Here's the drawing with two shaded views (mm, measured from the low corner). I have some questions. Coordinates: 2 decimals unless noted, no trailing zeros. Order: outer loops, then holes, each group sorted by start corner. A loop starts at its lowest first (then second) coordinate and runs counter-clockwise, first axis right, second up. Notation, with made-up numbers: (44, -22.5) -> (100, -22.5) arc R25 cw to (100, 1.5) -> close; hole circle Ø6 at (66.5, -24). An arc over 180 degrees is marked (long way). Return JSON: item names as keys, results as strings. Group by question number.
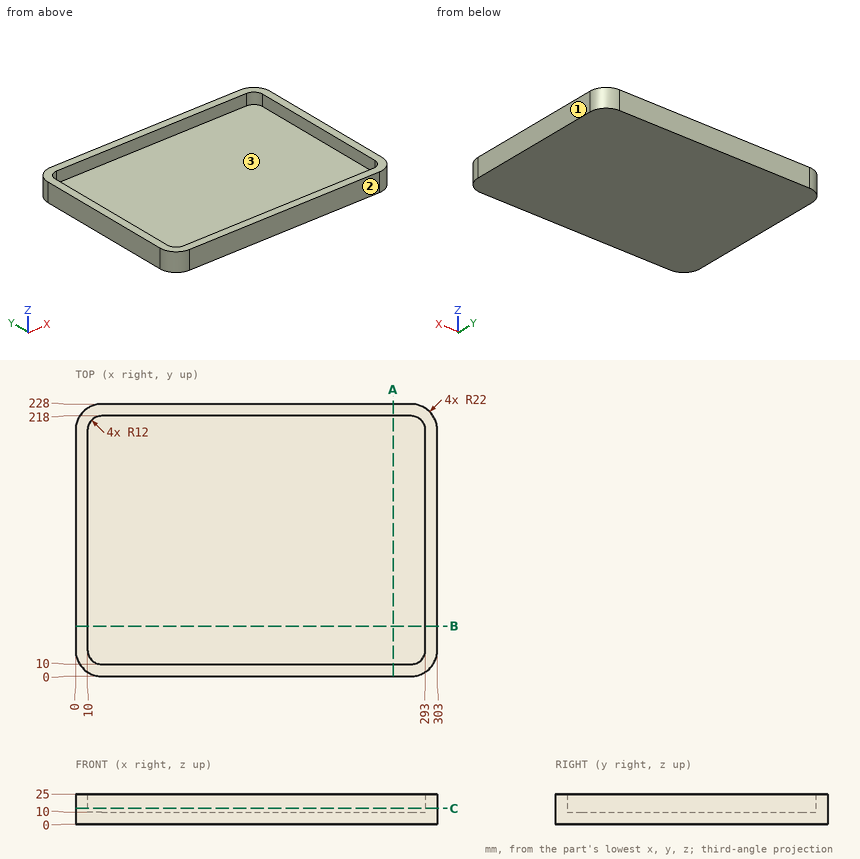
Q1. I'm going to push a flat-ended pin straight in: pin 1 Ø1.5 at (x, z) = (235, 11.5) entering from -Y. Where does the tip first touch, or does it pass through?
Q2. I need wall thicknesses on line 1 along Y through (x, z) = (181, 23.5); line 2 along X through (y, z) = (61.5, 11.5); line 3 along Z through (x, y) = (272, 66.5). Which ranges of each line are inside material? Lowest first, please. Write a range as from..to.
Q3. I want a section at A-A on x = 266. Please give me the cut outline in (y, z), and give its area (3 significant figures).
Q4. We'd pull the mould along X, two halves only. Please class the marked faces 1, 2 and 3: pulls with the +X half, pulls with the -X half, needs draft (parallel to the pull), parting line crosses it, or undercut.
Q5. I want a section at C-C on z = 13.25. Please give me the cut outline in (x, y), and give its area (3 significant figures).
Q6. I want a section at B-B on y = 42. Please give me the cut outline in (x, z).
Response values:
{
 "1": {"pin 1": "stops at y = 0"},
 "2": {"line 1": "y = 0..10, 218..228", "line 2": "x = 0..10, 293..303", "line 3": "z = 0..10"},
 "3": {"outline": "(0, 0) -> (228, 0) -> (228, 25) -> (218, 25) -> (218, 10) -> (10, 10) -> (10, 25) -> (0, 25) -> close", "area": "2,580 mm²"},
 "4": {"face 1": "pulls with the +X half", "face 2": "needs draft", "face 3": "undercut"},
 "5": {"outline": "(0, 22) arc R22 ccw to (22, 0) -> (281, 0) arc R22 ccw to (303, 22) -> (303, 206) arc R22 ccw to (281, 228) -> (22, 228) arc R22 ccw to (0, 206) -> close; hole (10, 22) arc R12 ccw to (22, 10) -> (281, 10) arc R12 ccw to (293, 22) -> (293, 206) arc R12 ccw to (281, 218) -> (22, 218) arc R12 ccw to (10, 206) -> close", "area": "9,930 mm²"},
 "6": {"outline": "(0, 0) -> (303, 0) -> (303, 25) -> (293, 25) -> (293, 10) -> (10, 10) -> (10, 25) -> (0, 25) -> close"}
}
